Verification items for the finished model (mm, model axes). Face numbers are marked on the shaded views. Give positions to 0.01 mm unless a question says otherwise; leave off trailing zeros. Loops run counter-clockwise (first coordinate to the right, second up) from the corner with the lowest first, then second, coordinate; pieces in that order, holes last. Notation, with made-up numbers: M 67.5,6 L 107.5,6 A13 ccw 107.5,21 Z; hole C 63.25,89 d3. An arc over 180 degrees is marked long. Write each question's results on one line, items separated by ' | '. Start each with the question number.
Solid Edge part; units mm, degrees
sketch "Sketch1" plane through (0, 0, -10) normal (0, 0, 1) x (1, 0, 0)
  line L0 (0, 4) -> (0, 40)
  line L1 (0, 40) -> (10, 40)
  line L2 (10, 40) -> (10, 0)
  line L3 (10, -40) -> (10, 0)
  line L4 (0, -40) -> (10, -40)
  line L5 (0, -4) -> (0, -40)
  arc A0 (0, -4) -> (0, 4) centre (0, 0) ccw
extrude "ExtrudedProtrusion_1" add sketch "Sketch1" along normal mid plane 16
sketch "Sketch2" plane through (0, 21, -10) normal (-1, 0, 0) x (0, 0, 1)
  circle A0 centre (0, 8.4449) radius 4.2
  circle A1 centre (0, -50.4449) radius 4.2
extrude "Cutout1" cut sketch "Sketch2" against normal through all
sketch "Sketch3" plane through (0, 21, -10) normal (-1, 0, 0) x (0, 0, 1)
  circle A0 centre (0, -14) radius 2.2
extrude "Cutout2" cut sketch "Sketch3" against normal through all
mirror "Mirror1" about plane through (0, 0, 0) normal (0, -1, 0) of "Cutout2"
sketch "Sketch4" plane through (10, 0, -10) normal (1, 0, 0) x (0, 1, 0)
  line L0 (0, 8) -> (-38, 8)
  line L1 (-38, 8) -> (-38, -14.4218)
extrude "Cutout4" cut sketch "Sketch4" against normal through all material side at (10, -19, -1.95)
mirror "Mirror2" about plane through (0, 0, 0) normal (0, -1, 0) of "Cutout4"
chamfer "Chamfer_1" distance 4 angle 45 4 edges at (5, -38, -2) (5, -38, -18) (5, 38, -2) (5, 38, -18)
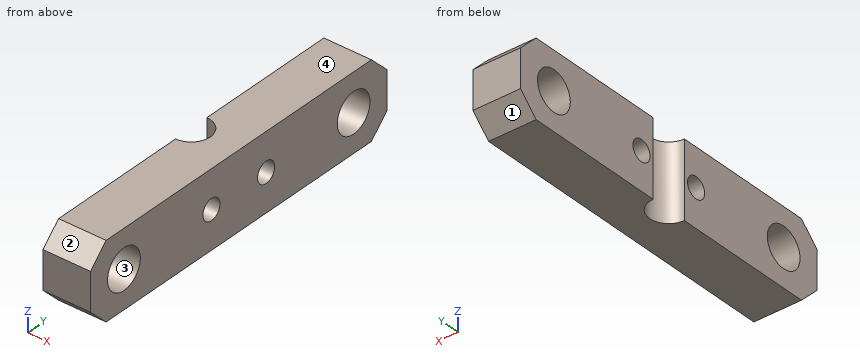
1. Release check for a two-part mould opening along Y. For the marked faces 1, 2, 3 and 4 record: released by +Y, released by -Y, zero draft, split by the parting line, or undercut.
2. Section check A-A, the plane y = 7. Record the boundary of the cut face in (x, z).
3. Thickness scan on probe 1 along Y at (x, z) = (8.25, -9.75); probe 2 along Y at (x, z) = (8.25, -10); probe 3 along Z at (x, y) = (7.5, -7). Record the ranges inside material, lowest first.
4. Section check B-B, the plane z = -10. Record the boundary of the cut face in (x, y).
5. Section check D-D, the plane z = -5. Record the boundary of the cut face in (x, y), plus the area to 3 significant figures.
6. Section check C-C, the plane x = 1.5. Record the boundary of the cut face in (y, z), plus the area to 3 significant figures.
Filled sheet:
1) face 1: released by +Y | face 2: released by -Y | face 3: undercut | face 4: zero draft
2) outline: M 0,-18 L 10,-18 L 10,-12.2 L 0,-12.2 Z; M 0,-7.8 L 10,-7.8 L 10,-2 L 0,-2 Z
3) probe 1: -38 to -33.64, -25.25 to -9.19, -4.81 to 4.81, 9.19 to 25.25, 33.64 to 38 | probe 2: -38 to -33.64, -25.24 to -9.2, -4.8 to 4.8, 9.2 to 25.24, 33.64 to 38 | probe 3: -18 to -12.2, -7.8 to -2
4) outline: M 0,-38 L 10,-38 L 10,-33.64 L 0,-33.64 Z; M 0,-25.24 L 10,-25.24 L 10,-9.2 L 0,-9.2 Z; M 0,-4.8 L 10,-4.8 L 10,4.8 L 0,4.8 L 0,4 A4 cw 0,-4 Z; M 0,9.2 L 10,9.2 L 10,25.24 L 0,25.24 Z; M 0,33.64 L 10,33.64 L 10,38 L 0,38 Z
5) outline: M 0,-37 L 10,-37 L 10,37 L 0,37 L 0,4 A4 cw 0,-4 Z | area: 715 mm2
6) outline: M -38,-14 L -34,-18 L -3.71,-18 L -3.71,-2 L -34,-2 L -38,-6 Z; M 3.71,-18 L 34,-18 L 38,-14 L 38,-6 L 34,-2 L 3.71,-2 Z; hole C -29.44,-10 d8.4; hole C -7,-10 d4.4; hole C 7,-10 d4.4; hole C 29.44,-10 d8.4 | area: 924 mm2
